from build123d import *

# Parameters (mm, degrees)
SKETCH_W         = 180
SKETCH_H         = 90
PAD_DEPTH        = 5
SKETCH001_R      = 37.5
POCKET_DEPTH     = 5
HOLE_D           = 4.4
HOLE_DEPTH       = 25
HOLE_CBORE_D     = 8
HOLE_CBORE_DEPTH = 2.4
SKETCH003_W      = 180
SKETCH003_H      = 90
SKETCH003_W_2    = 174
SKETCH003_H_2    = 84
PAD001_DEPTH     = 50


with BuildPart() as part:
    # Sketch → Pad (new body)
    with BuildSketch(Plane.XZ):
        Rectangle(SKETCH_W, SKETCH_H)
    extrude(amount=PAD_DEPTH)

    # Sketch001 (on Face6 of Pad) → Pocket (cut)
    with BuildSketch(Plane.XZ.offset(5)):
        with Locations((-42.872203, 0)):
            Circle(SKETCH001_R)
        with Locations((42.872203, 0)):
            Circle(SKETCH001_R)
    extrude(amount=-POCKET_DEPTH, mode=Mode.SUBTRACT)

    # Hole
    with Locations(Plane.XZ.offset(5)):
        with Locations((-78.622203, 35.75), (-7.122203, 35.75), (-78.622203, -35.75), (-7.122203, -35.75), (7.122203, 35.75), (78.622203, 35.75), (78.622203, -35.75), (7.122203, -35.75)):
            CounterBoreHole(HOLE_D / 2, HOLE_CBORE_D / 2, HOLE_CBORE_DEPTH, depth=HOLE_DEPTH)

    # Sketch003 (on Face5 of Pad) → Pad001 (join)
    with BuildSketch(Plane(origin=(0, 0, 0), x_dir=(1, 0, 0), z_dir=(0, 1, 0))):
        Rectangle(SKETCH003_W, SKETCH003_H)
        Rectangle(SKETCH003_W_2, SKETCH003_H_2, mode=Mode.SUBTRACT)
    extrude(amount=PAD001_DEPTH)


solid = part.part
The model under review builds one solid part; all positions refer to its coordinate system, in mm. A direction names the side the tool comes from. Give positions to 0.01 mm unless a question says otherwise; leave off trailing zeros. Order: outer loops, then holes, each group sorted by start corner. A loop starts at its lowest first (then second) coordinate and runs counter-clockwise, first axis right, second up. Notation, with made-up numbers: M 55,22.5 L 113,22.5 A6 cw 113,28.5 Z; hole C 13.25,50 d3. An arc over 180 degrees is marked long. Use one line per item in the form item = value. Start each with the question number.
Item 1: We need section A-A on y = 10.5. Give the boundary of the cut face in (x, z).
Item 2: The part is to be moulded in two halves that separate along Z. For faces 1 (the flat face through (-1, 22, 45)), 2 (the cylindrical face through (7.599, -1.282, 33.602)), 3 (the flat face through (90, 22, 1)), say which applies: pulls with the +Z half, pulls with the -Z half, needs draft (parallel to the pull), parting line crosses it, or undercut.
Item 3: We need section D-D on z = 17. Give the boundary of the cut face in (x, y), plus the area to 3 significant figures.
Item 4: For faces 4 (the flat face through (-1, 25, -42)), 5 (the cylindrical face through (-6.65, -1.28, -37.9)), 6 (the cylindrical face through (-7.643, -3.817, -31.784)), list the 3-axis set-ups (+Z, -Z, +X, -X, +Y, -Y) from which the entire face can be reached by the end or side of a thin tool; tool diameter is ignored.
Item 5: Insertion check: pin 1 Ø9 at (x, z) = (7.12, -35.75) entering from +Y; pin 2 Ø9 at (x, z) = (6.5, -35) entering from -Y; pin 3 Ø5.5 at (x, z) = (-78.62, -35.75) entering from -Y; pin 4 Ø3.5 at (x, z) = (-7.12, 35.75) entering from +Y. Each pin has a flat end and moves straight along its axis. Give the tip position at first contact, or say it passes through.
Item 6: We need section B-B on z = 0. Give the boundary of the cut face in (x, y).
Item 7: To check wall thickness, follow line 1 along Z through (x, y) = (5, 28.5); line 2 along X through (y, z) = (28, -34.5); line 3 along Y through (x, z) = (-73, 29.5). State the ranges of each line that lie inside material, in increasing order. Write a range as from..to.
Item 8: We need section C-C on x = 20.5. Give the boundary of the cut face in (y, z).
Completed:
q1.outline = M -90,-45 L 90,-45 L 90,45 L -90,45 Z; hole M -87,-42 L 87,-42 L 87,42 L -87,42 Z
q2.face_1 = pulls with the +Z half
q2.face_2 = undercut
q2.face_3 = needs draft
q3.outline = M -90,-5 L -76.3,-5 L -76.3,0 L -87,0 L -87,50 L -90,50 Z; M -9.45,-5 L 9.45,-5 L 9.45,0 L -9.45,0 Z; M 76.3,-5 L 90,-5 L 90,50 L 87,50 L 87,0 L 76.3,0 Z
q3.area = 531 mm²
q4.face_4 = +Y
q4.face_5 = +Y, -Y
q4.face_6 = -Y
q5.pin_1 = 0
q5.pin_2 = -5
q5.pin_3 = -2.6
q5.pin_4 = through
q6.outline = M -90,-5 L -80.37,-5 L -80.37,0 L -87,0 L -87,50 L -90,50 Z; M -5.37,-5 L 5.37,-5 L 5.37,0 L -5.37,0 Z; M 80.37,-5 L 90,-5 L 90,50 L 87,50 L 87,0 L 80.37,0 Z
q7.line_1 = -45..-42, 42..45
q7.line_2 = -90..-87, 87..90
q7.line_3 = -5..0
q8.outline = M -5,-45 L 50,-45 L 50,-42 L 0,-42 L 0,-30.1 L -5,-30.1 Z; M -5,30.1 L 0,30.1 L 0,42 L 50,42 L 50,45 L -5,45 Z
